Source: three-view drawing plus pictorial views. Frame: mm from the lowest corner of the part. Round coordinates to 2 decimals unless told otherwise and drop trailing zeros. Loops run counter-clockwise (first coordinate to the right, second up) from the corner with the lowest first, then second, coordinate; pieces in that order, holes last. Notation, with made-up numbers: (-7, 45) -> (50, 45) arc R20 cw to (50, 77) -> close; hole circle Ø8 at (9, 43.5). An arc over 180 degrees is marked (long way). Answer as a JSON object with one key per item and string values. Group by question number.
Item 1: Pin query (flat end, axial travel): pin 1 (3 mm diameter, centred on x = 11.635, y = 59, fed in from -Z); pin 2 (3.5 mm diameter, centred on x = 11.635, y = 144, fed in from -Z). Return the tip coordinate at first contact, or that it passes through.
Item 2: Material intervals for line 1 (X direction, y = 59, z = 2.85) (3 decimals); line 2 (X direction, y = 143, z = 4.65), sorted ascending. Write a range as [from, to].
Item 3: Section query A-A on y = 144. Return loops of the section in (x, z) (3 decimals).
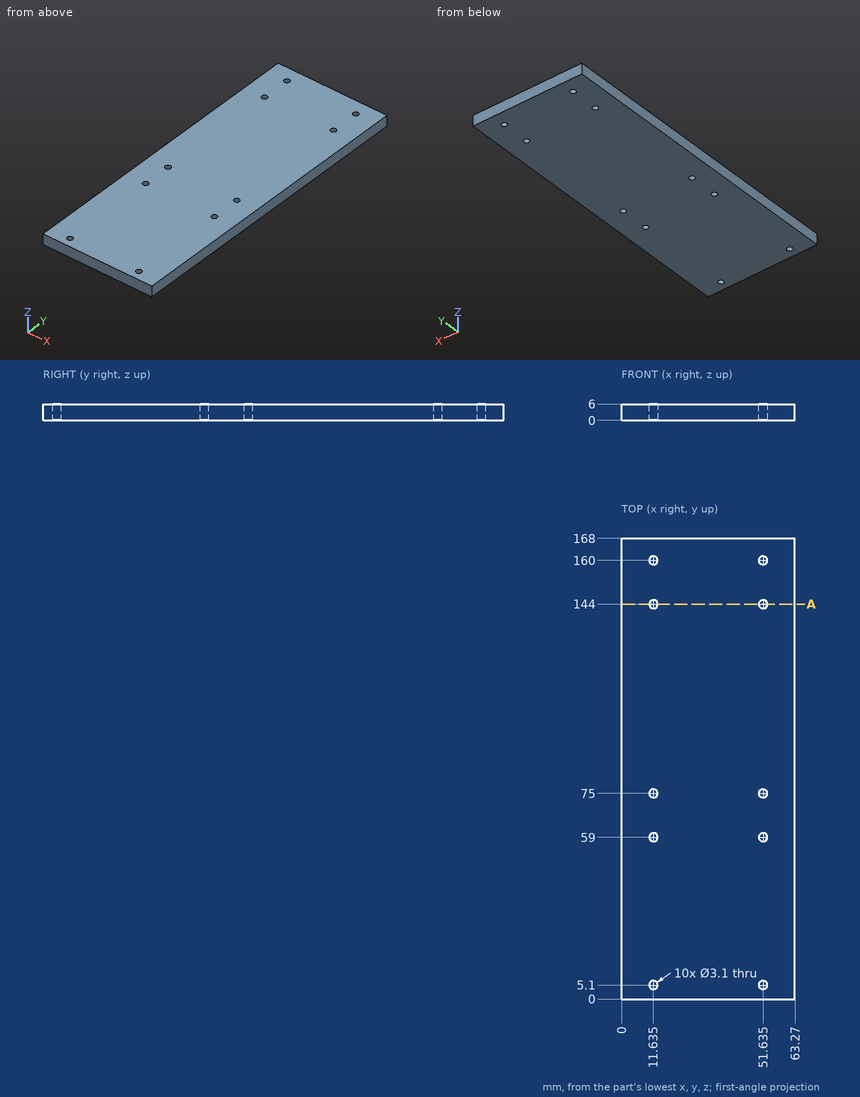
Solved:
{
 "1": {"pin 1": "through", "pin 2": "z = 0"},
 "2": {"line 1": "[0, 10.085], [13.185, 50.085], [53.185, 63.27]", "line 2": "[0, 10.45], [12.82, 50.45], [52.82, 63.27]"},
 "3": {"outline": "(0, 0) -> (10.085, 0) -> (10.085, 6) -> (0, 6) -> close; (13.185, 0) -> (50.085, 0) -> (50.085, 6) -> (13.185, 6) -> close; (53.185, 0) -> (63.27, 0) -> (63.27, 6) -> (53.185, 6) -> close"}
}
